Build history of the part. All positions in model axes, mm. A direction names the side the tool comes from. Round coordinates to 2 decimals unless told otherwise and drop trailing zeros. Loops run counter-clockwise (first coordinate to the right, second up) from the corner with the lowest first, then second, coordinate; pieces in that order, holes last. Notation, with made-up numbers: M 48,33 L 100,33 A8 ccw 100,37 Z; hole C -14.5,81 d10. An arc over 180 degrees is marked long. Use one line per item in the form item = value. Start each with the question number.
```python
from build123d import *

# Parameters (mm, degrees)
BOSS_EXTRUDE1_DEPTH            = 20
CUT_EXTRUDE7_REACH             = 109.052
SKETCH8_R                      = 3.1
FILLET1_R                      = 1
CUT_EXTRUDE8_REACH             = 119.729
SKETCH9_R                      = 2.1
CUT_EXTRUDE8_DIRECTION_2_REACH = 119.729
CUT_EXTRUDE9_REACH             = 127.729
CUT_EXTRUDE9_START             = -8
SKETCH10_R                     = 4
CUT_EXTRUDE10_REACH            = 127.729
CUT_EXTRUDE10_START            = -8
SKETCH11_R                     = 4
CUT_EXTRUDE11_DEPTH            = 5
CUT_EXTRUDE12_DEPTH            = 5


with BuildPart() as part:
    # Sketch1 → Boss-Extrude1 (new body)
    with BuildSketch(Plane.XY):
        with BuildLine():
            Line((-50, -15), (50, -15))
            Line((50, -15), (50, -11.808264258))
            ThreePointArc((50, -11.808264258), (49.644862571, -10.16054558), (48.64251158, -8.80541019))
            Line((48.64251158, -8.80541019), (28.393721051, 9.013525475))
            ThreePointArc((28.393721051, 9.013525475), (25.887843573, 12.40136395), (25, 16.520660644))
            Line((25, 16.520660644), (25, 82.520660644))
            ThreePointArc((25, 82.520660644), (22.071067812, 89.591728456), (15, 92.520660644))
            Line((15, 92.520660644), (-15, 92.520660644))
            ThreePointArc((-15, 92.520660644), (-22.071067812, 89.591728456), (-25, 82.520660644))
            Line((-25, 82.520660644), (-25, 16.520660644))
            ThreePointArc((-25, 16.520660644), (-25.887843573, 12.40136395), (-28.393721051, 9.013525475))
            Line((-28.393721051, 9.013525475), (-48.64251158, -8.80541019))
            ThreePointArc((-48.64251158, -8.80541019), (-49.644862571, -10.16054558), (-50, -11.808264258))
            Line((-50, -11.808264258), (-50, -15))
        make_face()
        with BuildLine():
            Line((-19, 10), (19, 10))
            ThreePointArc((19, 10), (19.707106781, 9.707106781), (20, 9))
            Line((20, 9), (20, -9))
            ThreePointArc((20, -9), (19.707106781, -9.707106781), (19, -10))
            Line((19, -10), (-19, -10))
            ThreePointArc((-19, -10), (-19.707106781, -9.707106781), (-20, -9))
            Line((-20, -9), (-20, 9))
            ThreePointArc((-20, 9), (-19.707106781, 9.707106781), (-19, 10))
        make_face(mode=Mode.SUBTRACT)
    extrude(amount=BOSS_EXTRUDE1_DEPTH)

    # Sketch8 → Cut-Extrude7 (cut, up to next)
    with BuildSketch(Plane(origin=(0, 0, 0), x_dir=(-1, 0, 0), z_dir=(0, 0, -1)), mode=Mode.PRIVATE) as cut_extrude7_sk1:
        with Locations((0, 77)):
            Circle(SKETCH8_R)
    cut_extrude7_tool1 = extrude(cut_extrude7_sk1.sketch, amount=-CUT_EXTRUDE7_REACH, mode=Mode.PRIVATE) & part.part
    add(cut_extrude7_tool1.solids().sort_by_distance((0, 77, 0))[0], mode=Mode.SUBTRACT)

    # Fillet1
    fillet1_edges = [part.edges().sort_by_distance(p)[0] for p in [
        (50, -13.404132129, 20),
        (-49.644862571, -10.16054558, 0),
        (-38.518116315, 0.104057643, 0),
        (49.644862571, -10.16054558, 20),
        (-25.887843573, 12.40136395, 0),
        (-25, 49.520660644, 0),
        (-22.071067812, 89.591728456, 0),
        (0, 92.520660644, 0),
        (22.071067812, 89.591728456, 0),
        (25, 49.520660644, 0),
        (25.887843573, 12.40136395, 0),
        (38.518116315, 0.104057643, 20),
        (38.518116315, 0.104057643, 0),
        (49.644862571, -10.16054558, 0),
        (50, -13.404132129, 0),
        (-50, -13.404132129, 0),
        (25.887843573, 12.40136395, 20),
        (25, 49.520660644, 20),
        (22.071067812, 89.591728456, 20),
        (0, 92.520660644, 20),
        (-22.071067812, 89.591728456, 20),
        (-25, 49.520660644, 20),
        (-25.887843573, 12.40136395, 20),
        (-50, -13.404132129, 20),
        (-38.518116315, 0.104057643, 20),
        (-49.644862571, -10.16054558, 20),
    ]]
    fillet(fillet1_edges, radius=FILLET1_R)

    # Sketch9 → Cut-Extrude8 (cut, up to next)
    with BuildSketch(Plane.ZY.offset(-20), mode=Mode.PRIVATE) as cut_extrude8_sk1:
        with Locations(Location((10, 0, 0), (0, 0, 90))):
            Circle(SKETCH9_R)
    cut_extrude8_tool1 = extrude(cut_extrude8_sk1.sketch, amount=-CUT_EXTRUDE8_REACH, mode=Mode.PRIVATE) & part.part
    add(cut_extrude8_tool1.solids().sort_by_distance((20, 0, 10))[0], mode=Mode.SUBTRACT)

    # Sketch9 → Cut-Extrude8 direction 2 (cut, up to next)
    with BuildSketch(Plane.ZY.offset(-20), mode=Mode.PRIVATE) as cut_extrude8_direction_2_sk1:
        with Locations(Location((10, 0, 0), (0, 0, 90))):
            Circle(SKETCH9_R)
    cut_extrude8_direction_2_tool1 = extrude(cut_extrude8_direction_2_sk1.sketch, amount=CUT_EXTRUDE8_DIRECTION_2_REACH, mode=Mode.PRIVATE) & part.part
    add(cut_extrude8_direction_2_tool1.solids().sort_by_distance((20, 0, 10))[0], mode=Mode.SUBTRACT)

    # Cut-Extrude9: up to this plane
    cut_extrude9_end = Plane(origin=(48.64251158, -8.80541019, 20), z_dir=(-0.660627894892025, -0.750713516922755, 0))
    # Sketch10 → Cut-Extrude9 (cut, up to the surface)
    with BuildSketch(Plane.ZY.offset(-20).offset(CUT_EXTRUDE9_START), mode=Mode.PRIVATE) as cut_extrude9_sk1:
        with Locations(Location((10, 0, 0), (0, 0, 270))):
            Circle(SKETCH10_R)
    cut_extrude9_tool1 = split(extrude(cut_extrude9_sk1.sketch, amount=-CUT_EXTRUDE9_REACH, mode=Mode.PRIVATE), bisect_by=cut_extrude9_end, keep=Keep.BOTH, mode=Mode.PRIVATE)
    add(cut_extrude9_tool1.solids().sort_by_distance((28, 0, 10))[0], mode=Mode.SUBTRACT)

    # Cut-Extrude10: up to this plane
    cut_extrude10_end = Plane(origin=(-48.64251158, -8.80541019, 20), z_dir=(0.6606278948920247, -0.7507135169227553, 0))
    # Sketch11 → Cut-Extrude10 (cut, up to the surface)
    with BuildSketch(Plane(origin=(-20, 0, 0), x_dir=(0, 0, -1), z_dir=(1, 0, 0)).offset(CUT_EXTRUDE10_START), mode=Mode.PRIVATE) as cut_extrude10_sk1:
        with Locations(Location((-10, 0, 0), (0, 0, 270))):
            Circle(SKETCH11_R)
    cut_extrude10_tool1 = split(extrude(cut_extrude10_sk1.sketch, amount=-CUT_EXTRUDE10_REACH, mode=Mode.PRIVATE), bisect_by=cut_extrude10_end, keep=Keep.BOTH, mode=Mode.PRIVATE)
    add(cut_extrude10_tool1.solids().sort_by_distance((-28, 0, 10))[0], mode=Mode.SUBTRACT)

    # Sketch12 → Cut-Extrude11 (cut)
    with BuildSketch(Plane(origin=(0, 0, 0), x_dir=(-1, 0, 0), z_dir=(0, 0, -1))):
        Polygon((5.773502692, 77), (2.886751346, 82), (-2.886751346, 82), (-5.773502692, 77), (-2.886751346, 72), (2.886751346, 72), align=None)
    extrude(amount=-CUT_EXTRUDE11_DEPTH, mode=Mode.SUBTRACT)

    # Sketch13 → Cut-Extrude12 (cut)
    with BuildSketch(Plane.XY.offset(20)):
        Polygon((5.773502692, 77), (2.886751346, 82), (-2.886751346, 82), (-5.773502692, 77), (-2.886751346, 72), (2.886751346, 72), align=None)
    extrude(amount=-CUT_EXTRUDE12_DEPTH, mode=Mode.SUBTRACT)


solid = part.part
```
Q1. Wall check: probe 1 along Y at (x, z) = (0, 7); probe 2 along Z at (x, y) = (-36, 0); probe 3 along Y at (x, z) = (7, 2.5). Give the ranges that are in metal, low to high.
Q2. Saw through at C-C (y = 50.5). Give the cut face in (x, z).
Q3. Saw through at D-D (z = 10). Give the number of separate pieces and of enclosed holes in the cut face, and give its area (3 significant figures).
Q4. Tool access for faces 1 (the face through (33.798, -3.815, 11.201)), 2 (the face through (-33.798, -3.815, 8.799)), 3 (the face through (0, 10, 10)), 4 (the face through (-25, 50, 10)), 5 (the face through (0, 82, 18)): list every direction of +Z, -Z, +X, -X, +Y, -Y with a clear straight run to the whole face (end or side of a thin tool).
Q5. Pull direction Y, two halves, no side cores. Call faces 6 (the face through (-1, 39, 20)), 7 (the face through (0, 72, 2)), 8 (the face through (-36.127, 2.209, 5.874)): pulls with the +Y half, pulls with the -Y half, needs draft (parallel to the pull), parting line crosses it, or undercut.
Q6. Saw through at B-B (z = 16.5). Give the cut face in (x, y).
Q7. Saw through at A-A (x = 0). Give the cut face in (y, z).
Q8. Drop flat-ended pins along their axis: P1, Ø5, axis at y = 0, z = 10, coming from the +X side; P2, Ø4, axis at y = 56, z = 16, coming from the +X side; P3, Ø12, axis at x = -25.5, z = 9, coming from the +Y side; P4, Ø3, axis at x = 39.5, y = 2, coming from the +Z side. Give the stop position or say it passes through.
Filled in:
q1.probe_1 = -15 to -10, 10 to 73.9, 80.1 to 92.52
q1.probe_2 = 0 to 6, 14 to 20
q1.probe_3 = -15 to -10, 10 to 92.52
q2.outline = M -25,1 A1 ccw -24,0 L 24,0 A1 ccw 25,1 L 25,19 A1 ccw 24,20 L -24,20 A1 ccw -25,19 Z
q3.separate_pieces = 2
q3.enclosed_holes = 1
q3.area = 5,070 mm²
q4.face_1 = +X
q4.face_2 = -X
q4.face_3 = +Z, -Z
q4.face_4 = +Z, -Z, -X, +Y
q4.face_5 = +Z
q5.face_6 = needs draft
q5.face_7 = undercut
q5.face_8 = pulls with the +Y half
q6.outline = M -50,-15 L 50,-15 L 50,-11.81 A4 ccw 48.64,-8.81 L 28.39,9.01 A10 cw 25,16.52 L 25,82.52 A10 ccw 15,92.52 L -15,92.52 A10 ccw -25,82.52 L -25,16.52 A10 cw -28.39,9.01 L -48.64,-8.81 A4 ccw -50,-11.81 Z; hole M -20,-9 A1 ccw -19,-10 L 19,-10 A1 ccw 20,-9 L 20,9 A1 ccw 19,10 L -19,10 A1 ccw -20,9 Z; hole M -5.77,77 L -2.89,72 L 2.89,72 L 5.77,77 L 2.89,82 L -2.89,82 Z
q7.outline = M -15,0 L -10,0 L -10,20 L -15,20 Z; M 10,0 L 72,0 L 72,5 L 73.9,5 L 73.9,15 L 72,15 L 72,20 L 10,20 Z; M 80.1,5 L 82,5 L 82,0 L 91.52,0 A1 ccw 92.52,1 L 92.52,19 A1 ccw 91.52,20 L 82,20 L 82,15 L 80.1,15 Z
q8.P1 = 28
q8.P2 = 25
q8.P3 = 91.45
q8.P4 = through
